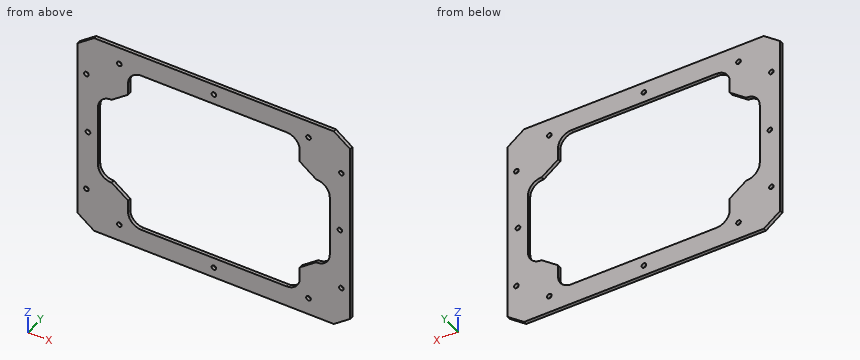
from build123d import *

# Parameters (mm, degrees)
BOSS_EXTRUDE1_DEPTH = 3.175
SKETCH2_R           = 2.159
CUT_EXTRUDE1_DEPTH  = 4.175


with BuildPart() as part:
    # Sketch1 → Boss-Extrude1 (new body)
    with BuildSketch(Plane(origin=(0, 0, 0), x_dir=(1, 0, 0), z_dir=(0, 1, 0))):
        Polygon((-111.686526805, 95.25), (-127, 83.918625912), (-127, -83.918625912), (-111.686526805, -95.25), (111.686526805, -95.25), (127, -83.918625912), (127, 83.918625912), (111.686526805, 95.25), align=None)
        with BuildLine():
            Line((-107.95, -28.564963508), (-107.95, 28.564963508))
            ThreePointArc((-107.95, 28.564963508), (-104.304650999, 37.365614506), (-95.504, 41.010963508))
            Line((-95.504, 41.010963508), (-95.25, 41.010963508))
            Line((-95.25, 41.010963508), (-79.936526805, 52.342337595))
            Line((-79.936526805, 52.342337595), (-79.936526805, 63.754))
            ThreePointArc((-79.936526805, 63.754), (-76.291177804, 72.554650999), (-67.490526805, 76.2))
            Line((-67.490526805, 76.2), (38.831798823, 76.2))
            Line((38.831798823, 76.2), (67.490526805, 76.2))
            ThreePointArc((67.490526805, 76.2), (76.291177804, 72.554650999), (79.936526805, 63.754))
            Line((79.936526805, 63.754), (79.936526805, 52.342337595))
            Line((79.936526805, 52.342337595), (95.25, 41.010963508))
            Line((95.25, 41.010963508), (95.504, 41.010963508))
            ThreePointArc((95.504, 41.010963508), (104.304650999, 37.365614506), (107.95, 28.564963508))
            Line((107.95, 28.564963508), (107.95, -28.564963508))
            ThreePointArc((107.95, -28.564963508), (104.304650999, -37.365614506), (95.504, -41.010963508))
            Line((95.504, -41.010963508), (95.25, -41.010963508))
            Line((95.25, -41.010963508), (79.936526805, -52.342337595))
            Line((79.936526805, -52.342337595), (79.936526805, -63.754))
            ThreePointArc((79.936526805, -63.754), (76.291177804, -72.554650999), (67.490526805, -76.2))
            Line((67.490526805, -76.2), (38.1, -76.2))
            Line((38.1, -76.2), (-67.490526805, -76.2))
            ThreePointArc((-67.490526805, -76.2), (-76.291177804, -72.554650999), (-79.936526805, -63.754))
            Line((-79.936526805, -63.754), (-79.936526805, -52.342337595))
            Line((-79.936526805, -52.342337595), (-95.25, -41.010963508))
            Line((-95.25, -41.010963508), (-95.504, -41.010963508))
            ThreePointArc((-95.504, -41.010963508), (-104.304650999, -37.365614506), (-107.95, -28.564963508))
        make_face(mode=Mode.SUBTRACT)
    extrude(amount=BOSS_EXTRUDE1_DEPTH)

    # Sketch2 → Cut-Extrude1 (cut, through all)
    with BuildSketch(Plane(origin=(0, 3.175, 0), x_dir=(1, 0, 0), z_dir=(0, 1, 0))):
        with Locations((-88.154790208, 79.461855841)):
            Circle(SKETCH2_R)
        with Locations((88.154790208, 79.461855841)):
            Circle(SKETCH2_R)
        with Locations((88.154790208, -79.461855841)):
            Circle(SKETCH2_R)
        with Locations((-88.154790208, -79.461855841)):
            Circle(SKETCH2_R)
        with Locations((-118.781736597, 56.799107666)):
            Circle(SKETCH2_R)
        with Locations((118.781736597, 56.799107666)):
            Circle(SKETCH2_R)
        with Locations((-118.781736597, -56.799107666)):
            Circle(SKETCH2_R)
        with Locations((118.781736597, -56.799107666)):
            Circle(SKETCH2_R)
        with Locations((0, -85.598)):
            Circle(SKETCH2_R)
        with Locations((0, 85.598)):
            Circle(SKETCH2_R)
        with Locations((-117.348, -0.020516524)):
            Circle(SKETCH2_R)
        with Locations((117.348, -0.020516524)):
            Circle(SKETCH2_R)
    extrude(amount=-CUT_EXTRUDE1_DEPTH, mode=Mode.SUBTRACT)


solid = part.part
Input: part model. Units: mm. Frame: model coordinates. Coordinates: 2 decimals unless noted, no trailing zeros. Order: outer loops, then holes, each group sorted by start corner. A loop starts at its lowest first (then second) coordinate and runs counter-clockwise, first axis right, second up.
1. Cut plane C-C, the plane y = 0.65. Count the separate pieces of the cut face and the enclosed holes in it, plus the area to 3 significant figures.
Checked values:
separate pieces: 1
enclosed holes: 13
area: 18,800 mm2
2. Ray query, line 1 along X through (y, z) = (1.3, 64.5); line 2 along Z through (x, y) = (-4, 2.7); line 3 along Z through (x, y) = (90, 2.6). Return the intervals inside material, ascending.
Checked values:
line 1: x = -127 to -79.91, 79.91 to 127
line 2: z = -95.25 to -76.2, 76.2 to 95.25
line 3: z = -95.25 to -80.58, -78.34 to -44.9, 44.9 to 78.34, 80.58 to 95.25
3. Cut plane A-A, the plane x = 21. Return loops of the section in (y, z) (3 decimals), plus the area to 3 significant figures.
Checked values:
outline: (0, -95.25) - (3.175, -95.25) - (3.175, -76.2) - (0, -76.2) - close; (0, 76.2) - (3.175, 76.2) - (3.175, 95.25) - (0, 95.25) - close
area: 121 mm2
4. Contact query for flat-ended pins moving along their axis: P1, Ø5.5, axis at x = 117.35, z = 0.02, coming from the -Y side; P2, Ø4, axis at x = 0, z = 85.598, coming from the -Y side. Output: stop coordinate, or through.
Checked values:
P1: stops at y = 0
P2: passes through
5. Cut plane B-B, the plane z = -8. Return loops of the section in (x, y) (3 decimals), plus the area to 3 significant figures.
Checked values:
outline: (-127, 0) - (-107.95, 0) - (-107.95, 3.175) - (-127, 3.175) - close; (107.95, 0) - (127, 0) - (127, 3.175) - (107.95, 3.175) - close
area: 121 mm2
